from build123d import *

# Parameters (mm, degrees)
F0_W     = 47.5
F0_H     = 35
F1_DEPTH = 17.5
F2_W     = 37.4171783071
F2_H     = 10.1249119453
F3_DEPTH = 35.001
F5_DEPTH = 10.0838216929
F7_DEPTH = 7.3760880547
F9_DEPTH = 7.3760880547


with BuildPart() as f1:
    # F0 (on Top) → F1 (new body)
    with BuildSketch(Plane.XY):
        with Locations((-23.6512488086, -2.9649846256)):
            Rectangle(F0_W, F0_H)
    extrude(amount=F1_DEPTH)

    # F2 (on face) → F3 (cut, through all)
    with BuildSketch(Plane.XZ.offset(20.4649846256)):
        with Locations((-18.6098379621, 12.4375440273)):
            Rectangle(F2_W, F2_H)
    extrude(amount=-F3_DEPTH, mode=Mode.SUBTRACT)

    # F4 (on face) → F5 (cut, through all)
    with BuildSketch(Plane.YZ.offset(-37.3184271157)):
        Polygon((9.5350153744, 17.5), (-15.4649846256, 17.5), (-12.9649846256, 13.1698729811), (7.0350153744, 13.1698729811), align=None)
    extrude(amount=-F5_DEPTH, mode=Mode.SUBTRACT)

    # F6 (on face) → F7 (cut, through all)
    with BuildSketch(Plane.XY.offset(7.3750880547)):
        Polygon((-22.5, -4.9646700483), (0.0987511914, -4.9646700483), (0.0987511914, 14.5350153744), (0, -0.9646700483), (-22.5, -0.9646700483), align=None)
    extrude(amount=-F7_DEPTH, mode=Mode.SUBTRACT)

    # F8 (on face) → F9 (cut, through all)
    with BuildSketch(Plane.XY.offset(7.3750880547)):
        Polygon((0.0987511914, -9.7249615937), (0.0987511914, -7.4646700483), (-12.4012488086, -20.4649846256), (0.0987511914, -20.4649846256), align=None)
        Polygon((-12.4012488086, 14.5350153744), (0.0159276115, 1.5352792135), (0.0987511914, 14.5350153744), align=None)
    extrude(amount=-F9_DEPTH, mode=Mode.SUBTRACT)


solid = f1.part
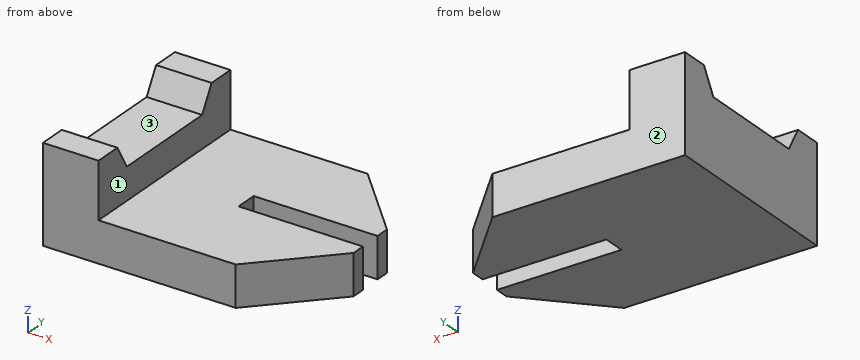
The listing builds one solid part. Answer for the finished solid, in the listing's coordinates (mm). Face numbers are marked on the shaded views. A direction names the side the tool comes from. Give positions to 0.01 mm unless a question says otherwise; leave off trailing zeros. Loops run counter-clockwise (first coordinate to the right, second up) from the corner with the lowest first, then second, coordinate; pieces in that order, holes last. Notation, with made-up numbers: (-27.75, 89) - (-4.75, 89) arc R11 ccw to (-4.75, 95) - close; hole circle Ø4 at (14, 80.25). An arc over 180 degrees is marked (long way). Write each question's results on one line, items separated by ' | '.
1. Which of the six approach directions +Z, -Z, +X, -X, +Y, -Y give full straight-line access (tool end or side, diameter ignored) to the marked faces 1, 2 and 3?
Resolved:
face 1: +Z, +X, +Y, -Y | face 2: +Z, -Z, +X, -X, +Y | face 3: +Z, +X, -X
2. Find section D-D, the plane z = 4.25. Write down the section's boundary in (x, y).
Resolved:
outline: (-47.4, -20.46) - (-12.4, -20.46) - (0.1, -7.46) - (0.1, -4.96) - (-22.5, -4.96) - (-22.5, -0.96) - (0, -0.96) - (0.02, 1.54) - (-12.4, 14.54) - (-47.4, 14.54) - close
3. Find section A-A, the plane z = 15.75. Write down the section's boundary in (x, y), then the cut area to 3 significant figures.
Resolved:
outline: (-47.4, -20.46) - (-37.32, -20.46) - (-37.32, -14.45) - (-47.4, -14.45) - close; (-47.4, 8.52) - (-37.32, 8.52) - (-37.32, 14.54) - (-47.4, 14.54) - close | area: 121 mm^2
4. Find section C-C, the plane x = -40. Write down the section's boundary in (y, z), then the cut area to 3 significant figures.
Resolved:
outline: (-20.46, 0) - (14.54, 0) - (14.54, 17.5) - (9.54, 17.5) - (7.04, 13.17) - (-12.96, 13.17) - (-15.46, 17.5) - (-20.46, 17.5) - close | area: 515 mm^2
5. Find section B-B, the plane x = -4. Write down the section's boundary in (y, z).
Resolved:
outline: (-11.73, 0) - (-4.96, 0) - (-4.96, 7.38) - (-11.73, 7.38) - close; (-0.96, 0) - (5.74, 0) - (5.74, 7.38) - (-0.96, 7.38) - close
6. Flat-ended cylindrical pins translate along their axes: P1, Ø3, axis at y = 1.5, z = 10.5, coming from the +X side; P2, Ø8, axis at x = -44.5, y = -7.5, coming from the +Z side; P3, Ø4.5, axis at y = -2.5, z = 5, coming from the +X side. Find the tip coordinate at first contact, or state that the pin passes through.
Resolved:
P1: stops at x = -37.32 | P2: stops at z = 13.17 | P3: stops at x = 0
7. Consider probe 1 along Y at (x, z) = (-16, 7.25); probe 2 along Z at (x, y) = (-13, 12); probe 3 along X at (y, z) = (2.5, 11.5). Determine where each line is inside the solid, lowest interval first. Write a range as from..to.
Resolved:
probe 1: y = -20.46..-4.96, -0.96..14.54 | probe 2: z = 0..7.38 | probe 3: x = -47.4..-37.32
